Read the model definition and answer for the solid it produces. Units are mm, in the model's axes. A direction names the side the tool comes from. Coordinates: 2 decimals unless noted, no trailing zeros. Loops run counter-clockwise (first coordinate to the right, second up) from the corner with the lowest first, then second, coordinate; pieces in that order, holes last. Notation, with made-up numbers: (63.25, -4) - (71.25, -4) arc R17 ccw to (71.25, 18) - close; hole circle Ø8 at (81, -20). An arc over 180 degrees is marked (long way). One line per item, written item: value. Start each with the question number.
from build123d import *

# Parameters (mm, degrees)
BOSS_EXTRU_1_DEPTH = 500
CONG_1_R           = 1
CHANFREIN1_DEPTH   = 500


with BuildPart() as part:
    # Esquisse1 → Boss.-Extru.1 (new body)
    with BuildSketch(Plane(origin=(0, 0, 0), x_dir=(0, 0, -1), z_dir=(1, 0, 0))):
        Polygon((0, 0), (5.5, 0), (5.5, -13), (29.5, -13), (29.5, 0), (35, 0), (35, -2), (31.5, -2), (31.5, -15), (3.5, -15), (3.5, -2), (0, -2), align=None)
    extrude(amount=BOSS_EXTRU_1_DEPTH)

    # Congé1
    cong_1_edges = [part.edges().sort_by_distance(p)[0] for p in [
        (250, 0, -5.5),
        (250, -13, -5.5),
        (250, -13, -29.5),
        (250, 0, -29.5),
        (250, -2, -31.5),
        (250, -15, -31.5),
        (250, -15, -3.5),
        (250, -2, -3.5),
    ]]
    fillet(cong_1_edges, radius=CONG_1_R)

    # Chanfrein1: read off the stored shape, not the designer's step
    # Chanfrein1 outline → Chanfrein1 (cut)
    with BuildSketch(Plane.YZ):
        with BuildLine():
            Line((-2.001381418, -2.552544532), (-1.002762836, 0))
            Line((-1.002762836, 0), (-2, 0))
            Line((-2, 0), (-2, -2.5))
            ThreePointArc((-2, -2.5), (-2.000345414, -2.526281344), (-2.001381418, -2.552544532))
        make_face()
        with BuildLine():
            Line((-1.002762836, -35), (-2.001381418, -32.447455468))
            ThreePointArc((-2.001381418, -32.447455468), (-2.000345414, -32.473718656), (-2, -32.5))
            Line((-2, -32.5), (-2, -35))
            Line((-2, -35), (-1.002762836, -35))
        make_face()
    extrude(amount=CHANFREIN1_DEPTH, mode=Mode.SUBTRACT)


solid = part.part
1) Flat-ended cylindrical pins translate along their axes: P1, Ø5.5, axis at x = 327.5, y = -10.5, coming from the +Z side; P2, Ø1.5, axis at x = 198.5, z = -14.5, coming from the +Y side; P3, Ø1, axis at y = -12, z = -25.5, coming from the +X side; P4, Ø5.5, axis at x = 313, y = -8.5, coming from the -Z side. Find the tip coordinate at first contact, or state that the pin passes through.
2) Determine the mould class of faces 4 (the flat face through (246, -15, -18)), 5 (the flat face through (246, -7, -29.5)), 6 (the flat face through (246, -9, -3.5)), 7 (the flat face through (246, -6, -5.5)) for opening direction Z: released by +Z, released by -Z, zero draft, split by the parting line, or undercut.
3) Section B-B, the plane x = 196.5 is taken. Determine the outline of the cut face in (y, z), and give its area (3 significant figures).
4) Section A-A, the plane y = -5.75 is taken. Determine the outline of the cut face in (x, z), and give its area (3 significant figures).
5) For faces 1 (the flat face through (246, -13, -17)), 2 (the flat face through (0, -14, -18)), 3 (the flat face through (246, -8, -31.5)), determine the directions among +Z, -Z, +X, -X, +Y, -Y from which every point of the face is accessible in a straight line to the end or side of a thin tool.
6) Section C-C, the plane z = -22.5 is taken. Determine the outline of the cut face in (x, y), and give its area (3 significant figures).
7) Straight lines are drawn through the part: L1, parallel to Z at x = 364, y = -3.75; L2, parallel to Y at x = 79, z = -21; L3, parallel to Z at x = 238.5, y = -2.5. For each, find the intervals that lie inside material, in ascending order.
Answer below:
1. P1: z = -3.5
1. P2: y = -13
1. P3: through
1. P4: z = -31.5
2. face 4: zero draft
2. face 5: undercut
2. face 6: released by +Z
2. face 7: undercut
3. outline: (-15, -30.5) arc R1 ccw to (-14, -31.5) - (-3, -31.5) arc R1 cw to (-2, -32.45) - (-1, -35) - (0, -35) - (0, -30.5) arc R1 ccw to (-1, -29.5) - (-12, -29.5) arc R1 cw to (-13, -28.5) - (-13, -6.5) arc R1 cw to (-12, -5.5) - (-1, -5.5) arc R1 ccw to (0, -4.5) - (0, 0) - (-1, 0) - (-2, -2.55) arc R1 cw to (-3, -3.5) - (-14, -3.5) arc R1 ccw to (-15, -4.5) - close
3. area: 119 mm2
4. outline: (0, -31.5) - (500, -31.5) - (500, -29.5) - (0, -29.5) - close; (0, -5.5) - (500, -5.5) - (500, -3.5) - (0, -3.5) - close
4. area: 2,000 mm2
5. face 1: +X, -X, +Y
5. face 2: +Z, -Z, -X, +Y, -Y
5. face 3: -Z, +X, -X, -Y
6. outline: (0, -15) - (500, -15) - (500, -13) - (0, -13) - close
6. area: 1,000 mm2
7. L1: -31.5 to -29.5, -5.5 to -3.5
7. L2: -15 to -13
7. L3: -31.63 to -29.5, -5.5 to -3.37
